Build history of the part. All positions in model axes, mm. Face numbers are marked on the shaded views. A direction names the side the tool comes from. Round coordinates to 2 decimals unless told otherwise and drop trailing zeros. Write each loop counter-clockwise with the first axis right and the second up, starting at its lowest first coordinate (ties: lowest second). Pieces come first, ordered by that corner, then holes. Notation, with made-up numbers: (51.5, 56.5) -> (72.5, 56.5) arc R16 ccw to (72.5, 86.5) -> close; hole circle Ø1 at (-37.5, -20). An arc over 180 degrees is marked (long way). Answer in a Markdown table with one row per item.
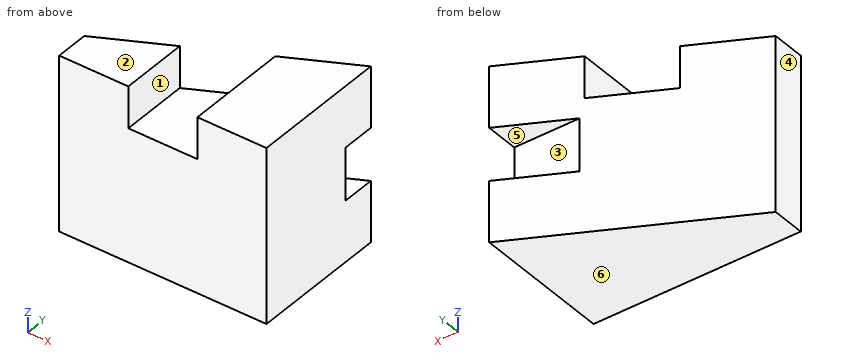
```python
from build123d import *

# Parameters (mm, degrees)
BOSS_EXTRUDE1_DEPTH = 63
CUT_EXTRUDE1_DEPTH  = 15
SKETCH6_W           = 19
SKETCH6_H           = 12
CUT_EXTRUDE3_DEPTH  = 25


with BuildPart() as part:
    # Sketch1 → Boss-Extrude1 (new body)
    with BuildSketch(Plane.XY):
        Polygon((75, 0), (0, 0), (0, 12), (75, 50), align=None)
    extrude(amount=BOSS_EXTRUDE1_DEPTH)

    # Sketch2 → Cut-Extrude1 (cut)
    with BuildSketch(Plane.XY.offset(63)):
        Polygon((25, 24.666666667), (25, 0), (50, 0), (50, 37.333333333), align=None)
    extrude(amount=-CUT_EXTRUDE1_DEPTH, mode=Mode.SUBTRACT)

    # Sketch6 → Cut-Extrude3 (cut)
    with BuildSketch(Plane(origin=(75, 0, 0), x_dir=(0, 0, -1), z_dir=(1, 0, 0))):
        with Locations((-31.5, 44)):
            Rectangle(SKETCH6_W, SKETCH6_H)
    extrude(amount=-CUT_EXTRUDE3_DEPTH, mode=Mode.SUBTRACT)


solid = part.part
```
Q1. Drop flat-ended pins along their axis: P1, Ø12, axis at y = 25.5, z = 56.5, coming from the -X side; P2, Ø8, axis at y = 38, z = 45.5, coming from the -X side; P3, Ø4, axis at y = 35.5, z = 54.5, coming from the -X side; P4, Ø8, axis at y = 41, z = 24, coming from the +X side. Give the stop position or say it passes through.
A:
| item | result |
|---|---|
| P1 | x = 14.8 |
| P2 | x = 43.42 |
| P3 | x = 50 |
| P4 | x = 75 |
Q2. Saw through at A-A on z = 51.5. Write the cut outline in (x, y).
A:
| item | result |
|---|---|
| outline | (0, 0) -> (25, 0) -> (25, 24.67) -> (0, 12) -> close; (50, 0) -> (75, 0) -> (75, 50) -> (50, 37.33) -> close |
Q3. Two-plate mould, pull along Z, no slides. Class the marked faces 4, 5 and 6: released by +Z, released by -Z, zero draft, split by the parting line, or undercut.
A:
| item | result |
|---|---|
| face 4 | zero draft |
| face 5 | undercut |
| face 6 | released by -Z |
Q4. Which spindle directions (+Z, -Z, +X, -X, +Y, -Y) get a long thin tool onto all of the face, cutting with end or side? Do the marked faces 1, 2 and 3. Say none if no direction does.
A:
| item | result |
|---|---|
| face 1 | +Z, +Y, -Y |
| face 2 | +Z, +X, -X, +Y, -Y |
| face 3 | +X, -X, +Y |
Q5. Saw through at D-D on z = 32.5. Write the cut outline in (x, y).
A:
| item | result |
|---|---|
| outline | (0, 0) -> (75, 0) -> (75, 38) -> (51.32, 38) -> (0, 12) -> close |
Q6. Saw through at B-B on y = 43.5. Write the cut outline in (x, z), plus the area to 3 significant figures.
A:
| item | result |
|---|---|
| outline | (62.17, 0) -> (75, 0) -> (75, 22) -> (62.17, 22) -> close; (62.17, 41) -> (75, 41) -> (75, 63) -> (62.17, 63) -> close |
| area | 564 mm² |
Q7. Wall check: line 1 (X direction, y = 4.5, z = 60); line 2 (Z direction, x = 65, y = 43.5); line 3 (X direction, y = 28, z = 49). Give the ranges that are in metal, low to high. Write a range as [from, to].
A:
| item | result |
|---|---|
| line 1 | [0, 25], [50, 75] |
| line 2 | [0, 22], [41, 63] |
| line 3 | [50, 75] |
Q8. Saw through at C-C on x = 69. Write the cut outline in (y, z).
A:
| item | result |
|---|---|
| outline | (0, 0) -> (46.96, 0) -> (46.96, 22) -> (38, 22) -> (38, 41) -> (46.96, 41) -> (46.96, 63) -> (0, 63) -> close |
